Check sheet for the modelled part. Datum: model origin and axes. Units: mm. Give positions to 0.01 mm unless a question says otherwise; leave off trailing zeros. Loops run counter-clockwise (first coordinate to the right, second up) from the corner with the lowest first, then second, coordinate; pieces in that order, holes last. Notation, with made-up numbers: (23, 25) - (37, 25) arc R27 cw to (37, 50) - close; hole circle Ø4 at (39, 16). An arc over 180 degrees is marked (long way). Use CSV: the item, a comma, the result in double quotes.
from build123d import *

# Parameters (mm, degrees)
F0_R     = 20
F1_DEPTH = 2.3
F2_R     = 10
F3_DEPTH = 2.301
F5_DEPTH = 6


with BuildPart() as f1:
    # F0 (on Top) → F1 (new body)
    with BuildSketch(Plane.XY):
        Circle(F0_R)
        Polygon((0, 4.1569219382), (3.6, 2.0784609691), (3.6, -2.0784609691), (0, -4.1569219382), (-3.6, -2.0784609691), (-3.6, 2.0784609691), align=None, mode=Mode.SUBTRACT)
    extrude(amount=F1_DEPTH)

    # F2 (on Top) → F3 (cut, through all)
    with BuildSketch(Plane.XY):
        with Locations((-20.8224465161, 16.605346988)):
            Circle(F2_R)
        with Locations((-25.9651661051, -5.926379725)):
            Circle(F2_R)
        with Locations((-11.5555860241, -23.9954216289)):
            Circle(F2_R)
        with Locations((11.5555860241, -23.9954216289)):
            Circle(F2_R)
        with Locations((25.9651661051, -5.926379725)):
            Circle(F2_R)
        with Locations((20.8224465161, 16.605346988)):
            Circle(F2_R)
    extrude(amount=F3_DEPTH, mode=Mode.SUBTRACT)

    # F4 (on Right) → F5 (cut, symmetric)
    with BuildSketch(Plane.YZ):
        Polygon((-20.0328639653, 3), (-20.0328639653, 0), (-14.5328639653, 3), align=None)
    extrude(amount=F5_DEPTH, both=True, mode=Mode.SUBTRACT)


solid = f1.part
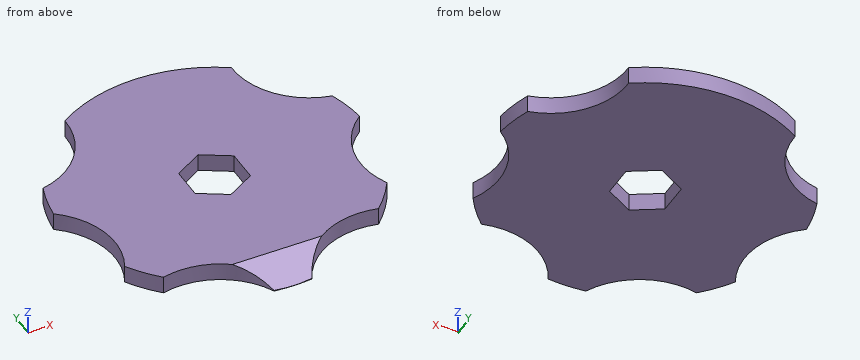
1. Sectioned sample at D-D, the plane y = -11. Record the boundary of the cut face in (x, z), and give its area (3 significant figures).
Completed:
outline,"(-16.7, 0) - (16.7, 0) - (16.7, 2.3) - (-16.7, 2.3) - close"
area,"76.8 mm²"
2. Scan lines: line 1 along Y through (x, z) = (0, 2); line 2 along X through (y, z) = (3, 1.7); line 3 along X through (y, z) = (-2.5, 2.25). Record each from-to range of solid material in increasing order.
Completed:
line 1,"y = -16.37 to -4.16, 4.16 to 20"
line 2,"x = -19.77 to -2, 2 to 19.77"
line 3,"x = -16.57 to -2.87, 2.87 to 16.57"
3. Sectioned sample at C-C, the plane z = 1.2. Record the boundary of the cut face in (x, y), and give its area (3 significant figures).
Completed:
outline,"(-19.9, 2.02) arc R10 cw to (-17.05, -10.46) arc R20 ccw to (-13.99, -14.3) arc R10 cw to (-3.68, -17.83) - (3.68, -17.83) arc R10 cw to (13.99, -14.3) arc R20 ccw to (17.05, -10.46) arc R10 cw to (19.9, 2.02) arc R20 ccw to (18.8, 6.81) arc R10 cw to (10.82, 16.82) arc R20 ccw to (-10.82, 16.82) arc R10 cw to (-18.8, 6.81) arc R20 ccw to start; hole (-3.6, -2.08) - (0, -4.16) - (3.6, -2.08) - (3.6, 2.08) - (0, 4.16) - (-3.6, 2.08) - close"
area,"1,020 mm²"
4. Go/stop test with flat-tipped pins: pin 1 Ø1.2 at (y, z) = (-0.5, 1.5) entering from -X (3 decimals); pin 2 Ø5 at (x, y) = (-7, -15) entering from -Z. Record where each tip stops, or that it passes through.
Completed:
pin 1,"stops at x = -17.985"
pin 2,"stops at z = 0"
5. Sectioned sample at B-B, the plane x = 16.5. Record the boundary of the cut face in (y, z), and give its area (3 significant figures).
Completed:
outline,"(-11.3, 0) - (-9.15, 0) - (-9.15, 2.3) - (-11.3, 2.3) - close; (-2.7, 0) - (7.59, 0) - (7.59, 2.3) - (-2.7, 2.3) - close"
area,"28.6 mm²"
6. Sectioned sample at A-A, the plane y = -1.5. Record the boundary of the cut face in (x, z).
Completed:
outline,"(-17, 0) - (-3.6, 0) - (-3.6, 2.3) - (-17, 2.3) - close; (3.6, 0) - (17, 0) - (17, 2.3) - (3.6, 2.3) - close"
